from build123d import *

# Parameters (mm, degrees)
SKETCH_1_W      = 125.77
SKETCH_1_H      = 70
EXTRUDE_1_DEPTH = 2


with BuildPart() as part:
    # 草图1 → 凸台-拉伸1 (new body)
    with BuildSketch(Plane.XY):
        Rectangle(SKETCH_1_W, SKETCH_1_H)
        with BuildLine():
            Line((-52.885, -18), (52.885, -18))
            ThreePointArc((52.885, -18), (54.885, -20), (52.885, -22))
            Line((52.885, -22), (-52.885, -22))
            ThreePointArc((-52.885, -22), (-54.885, -20), (-52.885, -18))
        make_face(mode=Mode.SUBTRACT)
        with BuildLine():
            Line((-52.885, -10), (52.885, -10))
            ThreePointArc((52.885, -10), (54.885, -12), (52.885, -14))
            Line((52.885, -14), (-52.885, -14))
            ThreePointArc((-52.885, -14), (-54.885, -12), (-52.885, -10))
        make_face(mode=Mode.SUBTRACT)
        with BuildLine():
            Line((-52.885, -2), (52.885, -2))
            ThreePointArc((52.885, -2), (54.885, -4), (52.885, -6))
            Line((52.885, -6), (-52.885, -6))
            ThreePointArc((-52.885, -6), (-54.885, -4), (-52.885, -2))
        make_face(mode=Mode.SUBTRACT)
        with BuildLine():
            Line((-52.885, 6), (52.885, 6))
            ThreePointArc((52.885, 6), (54.885, 4), (52.885, 2))
            Line((52.885, 2), (-52.885, 2))
            ThreePointArc((-52.885, 2), (-54.885, 4), (-52.885, 6))
        make_face(mode=Mode.SUBTRACT)
        with BuildLine():
            Line((-52.885, 14), (52.885, 14))
            ThreePointArc((52.885, 14), (54.885, 12), (52.885, 10))
            Line((52.885, 10), (-52.885, 10))
            ThreePointArc((-52.885, 10), (-54.885, 12), (-52.885, 14))
        make_face(mode=Mode.SUBTRACT)
        with BuildLine():
            Line((-52.885, 22), (52.885, 22))
            ThreePointArc((52.885, 22), (54.885, 20), (52.885, 18))
            Line((52.885, 18), (-52.885, 18))
            ThreePointArc((-52.885, 18), (-54.885, 20), (-52.885, 22))
        make_face(mode=Mode.SUBTRACT)
        with BuildLine():
            Line((-52.885, 30), (52.885, 30))
            ThreePointArc((52.885, 30), (54.885, 28), (52.885, 26))
            Line((52.885, 26), (-52.885, 26))
            ThreePointArc((-52.885, 26), (-54.885, 28), (-52.885, 30))
        make_face(mode=Mode.SUBTRACT)
        with BuildLine():
            Line((-52.885, -26), (52.885, -26))
            ThreePointArc((52.885, -26), (54.885, -28), (52.885, -30))
            Line((52.885, -30), (-52.885, -30))
            ThreePointArc((-52.885, -30), (-54.885, -28), (-52.885, -26))
        make_face(mode=Mode.SUBTRACT)
    extrude(amount=EXTRUDE_1_DEPTH)


solid = part.part
Model file for the job. Use its own axes, mm. Round coordinates to 2 decimals unless told otherwise and drop trailing zeros. Loops run counter-clockwise (first coordinate to the right, second up) from the corner with the lowest first, then second, coordinate; pieces in that order, holes last. Notation, with made-up numbers: (71.5, 6.5) -> (113.5, 6.5) arc R26 cw to (113.5, 27.5) -> close; hole circle Ø4 at (20, -33). An arc over 180 degrees is marked (long way). Answer as CSV lines item,"result". Start each with the question number.
1) Slice it at B-B (x = 40). State how many separate pieces and enclosed holes the cut face has, plus the area to 3 significant figures.
2) Slice it at D-D (y = -3.5). List the corners of the cut face in (x, z) (1 decimal), plus the area to 3 significant figures.
3) Probe line 1 along X through (y, z) = (-4, 1.35) (3 decimals); line 2 along X through (y, z) = (3, 0.5) (3 decimals). List the from-to ranges inside material, lowest first.
4) Slice it at A-A (y = -28). List the corners of the cut face in (x, z) (3 decimals).
Filled in:
1,separate pieces,"9"
1,enclosed holes,"0"
1,area,"76.0 mm2"
2,outline,"(-62.9, 0) -> (-54.8, 0) -> (-54.8, 2) -> (-62.9, 2) -> close; (54.8, 0) -> (62.9, 0) -> (62.9, 2) -> (54.8, 2) -> close"
2,area,"32.3 mm2"
3,line 1,"x = -62.885 to -54.885, 54.885 to 62.885"
3,line 2,"x = -62.885 to -54.617, 54.617 to 62.885"
4,outline,"(-62.885, 0) -> (-54.885, 0) -> (-54.885, 2) -> (-62.885, 2) -> close; (54.885, 0) -> (62.885, 0) -> (62.885, 2) -> (54.885, 2) -> close"
